```python
from build123d import *

# Parameters (mm, degrees)
SKETCH1_W                      = 18
SKETCH1_H                      = 18
BOSS_EXTRUDE1_DEPTH            = 5.75
M2_CLEARANCE_HOLE1_D           = 2.4
M2_CLEARANCE_HOLE1_CSINK_D     = 2.45
M2_CLEARANCE_HOLE1_CSINK_ANGLE = 90
SKETCH5_W                      = 5.8
SKETCH5_H                      = 7
BOSS_EXTRUDE2_DEPTH            = 50
SKETCH6_R                      = 4.0625
CUT_EXTRUDE1_DEPTH             = 5.75
SKETCH7_R                      = 3.25
CUT_EXTRUDE2_DEPTH             = 5.75
FILLET1_R                      = 2
M2_CLEARANCE_HOLE2_D           = 2.4
M2_CLEARANCE_HOLE2_DEPTH       = 5.75
M2_CLEARANCE_HOLE2_TIP         = 0.721032743
SKETCH11_W                     = 5
SKETCH11_H                     = 7
SKETCH11_W_2                   = 7
SKETCH11_H_2                   = 4
BOSS_EXTRUDE3_DEPTH            = 5.75
SKETCH12_W                     = 5
SKETCH12_H                     = 7
SKETCH12_W_2                   = 7
SKETCH12_H_2                   = 4
BOSS_EXTRUDE4_DEPTH            = 5.75
FILLET2_R                      = 2
SKETCH15_R                     = 4.0625
SKETCH15_R_2                   = 0.75
BOSS_EXTRUDE5_DEPTH            = 5.75
SKETCH16_R                     = 2
SKETCH16_R_2                   = 0.75
BOSS_EXTRUDE6_DEPTH            = 25
SKETCH17_R                     = 5
SKETCH17_R_2                   = 1.5
CUT_EXTRUDE3_DEPTH             = 2.75
CHAMFER1_SIZE                  = 0.25
CHAMFER1_SIZE2                 = 0.297408065
FILLET3_R                      = 1


with BuildPart() as part:
    # Sketch1 → Boss-Extrude1 (new body)
    with BuildSketch(Plane(origin=(0, 0, 0), x_dir=(1, 0, 0), z_dir=(0, 1, 0))):
        Rectangle(SKETCH1_W, SKETCH1_H)
    boss_extrude1 = extrude(amount=BOSS_EXTRUDE1_DEPTH)

    # M2 Clearance Hole1 (through all)
    with Locations(Plane(origin=(0, 5.75, 0), x_dir=(1, 0, 0), z_dir=(0, 1, 0))):
        with Locations((-6, 6), (6, 6), (-6, -6), (6, -6)):
            CounterSinkHole(M2_CLEARANCE_HOLE1_D / 2, M2_CLEARANCE_HOLE1_CSINK_D / 2, counter_sink_angle=M2_CLEARANCE_HOLE1_CSINK_ANGLE)

    # Sketch5 → Boss-Extrude2 (add)
    with BuildSketch(Plane(origin=(0, 5.75, 0), x_dir=(1, 0, 0), z_dir=(0, 1, 0))):
        with Locations((-11.1, 0)):
            Rectangle(SKETCH5_W, SKETCH5_H)
        with Locations((11.1, 0)):
            Rectangle(SKETCH5_W, SKETCH5_H)
        Polygon((3.5, -7), (1.5, -7), (1.5, -7.5), (-1.5, -7.5), (-1.5, -7), (-3.5, -7), (-3.5, -9), (-3.5, -13), (3.5, -13), (3.5, -9), align=None)
    extrude(amount=BOSS_EXTRUDE2_DEPTH)

    # Sketch6 → Cut-Extrude1 (cut)
    with BuildSketch(Plane(origin=(0, 5.75, 0), x_dir=(1, 0, 0), z_dir=(0, 1, 0))):
        with Locations(Location((0, 0, 0), (0, 0, 270))):
            Circle(SKETCH6_R)
    extrude(amount=-CUT_EXTRUDE1_DEPTH, mode=Mode.SUBTRACT)

    # Mirror1: Boss-Extrude1 across plane
    add(boss_extrude1.mirror(Plane.ZX.offset(30.75)))

    # Sketch7 → Cut-Extrude2 (cut)
    with BuildSketch(Plane(origin=(0, 61.5, 0), x_dir=(1, 0, 0), z_dir=(0, 1, 0))):
        with Locations(Location((0, 0, 0), (0, 0, 270))):
            Circle(SKETCH7_R)
    extrude(amount=-CUT_EXTRUDE2_DEPTH, mode=Mode.SUBTRACT)

    # Fillet1
    fillet1_edges = [part.edges().sort_by_distance(p)[0] for p in [
        (9, 58.625, -9),
        (9, 58.625, 9),
        (-9, 58.625, 9),
        (-9, 58.625, -9),
        (9, 2.875, 9),
        (-9, 2.875, 9),
        (-9, 2.875, -9),
        (9, 2.875, -9),
    ]]
    fillet(fillet1_edges, radius=FILLET1_R)

    # M2 Clearance Hole2
    with Locations(Plane(origin=(0, 61.5, 0), x_dir=(1, 0, 0), z_dir=(0, 1, 0))):
        with Locations((-3.535533906, -3.535533906), (3.535533906, 3.535533906)):
            Hole(M2_CLEARANCE_HOLE2_D / 2, depth=M2_CLEARANCE_HOLE2_DEPTH)
            with Locations((0, 0, -(M2_CLEARANCE_HOLE2_DEPTH + M2_CLEARANCE_HOLE2_TIP / 2))):  # 118° drill point
                Cone(0, M2_CLEARANCE_HOLE2_D / 2, M2_CLEARANCE_HOLE2_TIP, mode=Mode.SUBTRACT)

    # Sketch11 → Boss-Extrude3 (add)
    with BuildSketch(Plane(origin=(0, 55.75, 0), x_dir=(1, 0, 0), z_dir=(0, 1, 0))):
        with Locations((-11.5, 0)):
            Rectangle(SKETCH11_W, SKETCH11_H)
        with Locations((11.5, 0)):
            Rectangle(SKETCH11_W, SKETCH11_H)
        with Locations((0, -11)):
            Rectangle(SKETCH11_W_2, SKETCH11_H_2)
    extrude(amount=BOSS_EXTRUDE3_DEPTH)

    # Sketch12 → Boss-Extrude4 (add)
    with BuildSketch(Plane.XZ.offset(-5.75)):
        with Locations((-11.5, 0)):
            Rectangle(SKETCH12_W, SKETCH12_H)
        with Locations((0, 11)):
            Rectangle(SKETCH12_W_2, SKETCH12_H_2)
        with Locations((11.5, 0)):
            Rectangle(SKETCH12_W, SKETCH12_H)
    extrude(amount=BOSS_EXTRUDE4_DEPTH)

    # Fillet2
    fillet2_edges = [part.edges().sort_by_distance(p)[0] for p in [
        (-14, 30.75, -3.5),
        (-14, 30.75, 3.5),
        (-3.5, 30.75, 13),
        (3.5, 30.75, 13),
        (14, 30.75, -3.5),
        (14, 30.75, 3.5),
    ]]
    fillet(fillet2_edges, radius=FILLET2_R)

    # Sketch15 → Boss-Extrude5 (add)
    with BuildSketch(Plane(origin=(0, 5.75, 0), x_dir=(1, 0, 0), z_dir=(0, 1, 0))):
        Circle(SKETCH15_R)
        with Locations(Location((0, 0, 0), (0, 0, 270))):
            Circle(SKETCH15_R_2, mode=Mode.SUBTRACT)
    extrude(amount=-BOSS_EXTRUDE5_DEPTH)

    # Sketch16 → Boss-Extrude6 (add)
    with BuildSketch(Plane.XZ):
        with Locations(Location((0, 0, 0), (0, 0, 270))):
            Circle(SKETCH16_R)
        with Locations(Location((0, 0, 0), (0, 0, 90))):
            Circle(SKETCH16_R_2, mode=Mode.SUBTRACT)
    extrude(amount=BOSS_EXTRUDE6_DEPTH)

    # Sketch17 → Cut-Extrude3 (cut)
    with BuildSketch(Plane(origin=(0, 5.75, 0), x_dir=(1, 0, 0), z_dir=(0, 1, 0))):
        with Locations(Location((0, 0, 0), (0, 0, 270))):
            Circle(SKETCH17_R)
        with Locations(Location((0, 0, 0), (0, 0, 270))):
            Circle(SKETCH17_R_2, mode=Mode.SUBTRACT)
    extrude(amount=-CUT_EXTRUDE3_DEPTH, mode=Mode.SUBTRACT)

    # Sketch19 → Cut-Revolve1 (revolve, cut)
    with BuildSketch(Plane.XY, mode=Mode.PRIVATE) as cut_revolve1_sk:
        Polygon((0, -25), (-1.5, -25), (0, -15), align=None)
    revolve(cut_revolve1_sk.sketch.rotate(Axis((0, -15, 0), (0, -1, 0)), 270), axis=Axis((0, -15, 0), (0, -1, 0)), mode=Mode.SUBTRACT)

    # Chamfer1
    chamfer1_edges = [part.edges().sort_by_distance(p)[0] for p in [
        (0, -25, -1.5),
    ]]
    chamfer1_side = [part.faces().sort_by_distance(p)[0] for p in [
        (0, -22.5, -1.125),
    ]]
    chamfer(chamfer1_edges, length=CHAMFER1_SIZE, length2=CHAMFER1_SIZE2, reference=chamfer1_side[0])

    # Fillet3
    # the kernel refuses this fillet: 1 mm, written as the material it takes off along each edge
    with BuildSketch(Plane(origin=(0, 5.75, 0), x_dir=(0, 0, 1), z_dir=(-1, 0, 0))) as fillet3_piece_1:
        with BuildLine():
            CenterArc((0.5, -0.968245837), FILLET3_R, 0, 75.522487814)
            Line((1.5, -0.968245837), (1.52, -0.968245837))
            Line((1.52, -0.968245837), (1.52, 0))
            Line((1.52, 0), (1.5, 0.02))
            ThreePointArc((1.5, 0.02), (1.125, 0.02), (0.755, 0.019364917))
            Line((0.755, 0.019364917), (0.75, 0))
        make_face()
    revolve(axis=Axis((0, 5.75, 0), (0, 1, 0)), mode=Mode.SUBTRACT)


solid = part.part
```
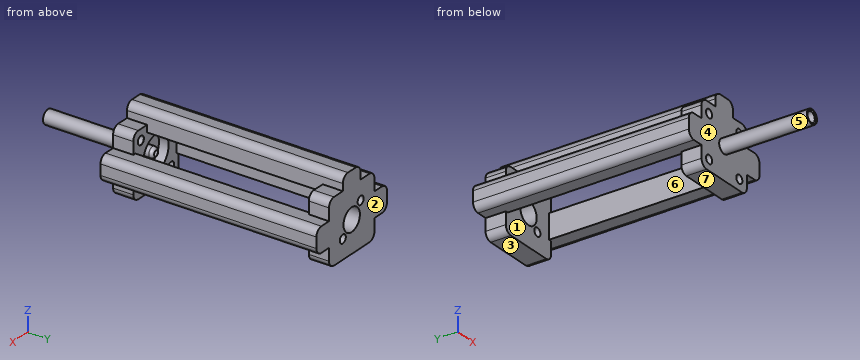
For this review, take the finished solid that the model builds, in its own axes (mm). Face numbers are marked on the shaded views. A direction names the side the tool comes from. Round coordinates to 2 decimals unless told otherwise and drop trailing zeros. Write each loop counter-clockwise with the first axis right and the second up, starting at its lowest first coordinate (ties: lowest second). Pieces come first, ordered by that corner, then holes. Notation, with made-up numbers: (75, 26.25) -> (118, 26.25) arc R21 ccw to (118, 53.25) -> close; hole circle Ø5 at (-30.5, 80.25). An arc over 180 degrees is marked (long way). Use one line per item in the form item = value.
1) Tool access review of the marked faces 5, 6 and 7: name each direction out of +Z, -Z, +X, -X, +Y, -Y from which nothing blocks a thin tool from reaching the whole face with its end or side.
Found:
face_5 = -Y
face_6 = +Z, -Z
face_7 = -Z, +X, -X, +Y, -Y
2) Take a section at A-A, the plane x = 6. Write out the cut boundary in (y, z) (3 decimals).
Found:
outline = (0, -9) -> (5.75, -9) -> (5.75, -7.225) -> (5.725, -7.2) -> (0, -7.2) -> close; (0, -4.8) -> (5.725, -4.8) -> (5.75, -4.775) -> (5.75, 4.775) -> (5.725, 4.8) -> (0, 4.8) -> close; (0, 7.2) -> (5.725, 7.2) -> (5.75, 7.225) -> (5.75, 9) -> (0, 9) -> close; (55.75, -9) -> (61.5, -9) -> (61.5, 9) -> (55.75, 9) -> close
3) Take a section at C-C, the plane y = 13. Write out the cut boundary in (x, z), and give its area (3 significant figures).
Found:
outline = (-14, -1.5) arc R2 ccw to (-12, -3.5) -> (-8.2, -3.5) -> (-8.2, 3.5) -> (-12, 3.5) arc R2 ccw to (-14, 1.5) -> close; (-3.5, 7) -> (-1.5, 7) -> (-1.5, 7.5) -> (1.5, 7.5) -> (1.5, 7) -> (3.5, 7) -> (3.5, 11) arc R2 ccw to (1.5, 13) -> (-1.5, 13) arc R2 ccw to (-3.5, 11) -> close; (8.2, -3.5) -> (12, -3.5) arc R2 ccw to (14, -1.5) -> (14, 1.5) arc R2 ccw to (12, 3.5) -> (8.2, 3.5) -> close
area = 117 mm2
4) Mouldability with a two-part tool opening along Y and no side actions: class the marked faces 1, 2, 3 and 4 as +Y half, -Y half, draft (parallel to the pull), parting line (faces both ways), or undercut.
Found:
face_1 = undercut
face_2 = +Y half
face_3 = draft
face_4 = -Y half
5) Take a section at D-D, the plane y = -6. Write out the cut boundary in (x, z).
Found:
outline = circle Ø4 at (0, 0); hole circle Ø1.5 at (0, 0)
6) To check wall thickness, follow L1, parallel to X at y = 3.45, z = 0; L2, parallel to X at y = 4.45, z = -6. State the ranges of each line that lie inside material, in increasing order. Write a range as from..to.
Found:
L1 = -14..-5, -1.5..-0.75, 0.75..1.5, 5..14
L2 = -9..-7.2, -4.8..4.8, 7.2..9
7) Take a section at B-B, the plane z = 6. Write out the cut boundary in (x, y) (3 decimals), and give its area (3 significant figures).
Found:
outline = (-9, 0) -> (-7.2, 0) -> (-7.2, 5.725) -> (-7.225, 5.75) -> (-9, 5.75) -> close; (-9, 55.75) -> (9, 55.75) -> (9, 61.5) -> (-9, 61.5) -> close; (-4.8, 0) -> (4.8, 0) -> (4.8, 5.725) -> (4.775, 5.75) -> (-4.775, 5.75) -> (-4.8, 5.725) -> close; (7.2, 0) -> (9, 0) -> (9, 5.75) -> (7.225, 5.75) -> (7.2, 5.725) -> close
area = 179 mm2
8) Clearance check with flat-ended pins moving along their axes: pin 1 (4 mm diameter, centred on x = 0, y = -4, fed in from +Z); pin 2 (1.8 mm diameter, centred on y = 59, z = 5, fed in from -X); pin 3 (4 mm diameter, centred on x = -4.5, y = 58, fed in from +Z). State where each tip first meets the part, or that it passes through.
Found:
pin_1 = 2
pin_2 = -9
pin_3 = 12.73
